Autodesk Inventor part; units mm, degrees
ref_plane "YZ Plane" through (0, 0, 0) normal (1, 0, 0) x (0, 1, 0)
ref_plane "XZ Plane" through (0, 0, 0) normal (0, 1, 0) x (-1, 0, 0)
ref_plane "XY Plane" through (0, 0, 0) normal (0, 0, 1) x (1, 0, 0)
sketch "Sketch1" plane through (0, 0, 0) normal (0, 0, 1) x (1, 0, 0)
  line L0 (9.525, -12.7) -> (-9.525, -12.7)
  line L1 (-9.525, -12.7) -> (-9.525, 12.7)
  line L2 (-9.525, 12.7) -> (9.525, 12.7)
  line L3 (9.525, 12.7) -> (9.525, -12.7)
  line L4 (9.525, -12.7) -> (-9.525, 12.7) construction
  line L5 (-9.525, -12.7) -> (9.525, 12.7) construction
  line L6 (-9.525, 12.7) -> (0, 12.7)
  line L7 (0, 12.7) -> (0, -50.8)
  line L8 (0, -50.8) -> (-9.525, -50.8)
  line L9 (-9.525, -50.8) -> (-9.525, 12.7)
  line L10 (-9.525, -50.8) -> (9.525, -43.8664)
  line L11 (-9.525, -50.8) -> (10.7476, -50.8) construction
  line L12 (9.525, -43.8664) -> (0, -35.8739)
  point P0 (0, 0)
  point P1 (0, -12.7)
  dimension "d0" = 19.05
  dimension "d1" = 25.4
  dimension "d2" = 63.5
  dimension "d3" = 20
  dimension "d4" = 60
extrude "Extrusion1" add sketch "Sketch1" along normal blind 3.175 contours L0 L7 L2 L3 | L7 L10 L9 L0 | L0 L1 L2 L7 | L12 L10 L7
sketch "Sketch2" plane through (0, 0, 3.175) normal (0, 0, 1) x (1, 0, 0)
  line L0 (-9.525, 12.7) -> (-9.525, -50.8) construction
  line L1 (-9.525, 0) -> (9.525, 0) construction
  line L2 (9.525, -12.7) -> (9.525, 12.7) construction
  line L3 (9.525, 12.7) -> (-9.525, 12.7) construction
  line L4 (0, -35.8739) -> (0, -12.7) construction
  line L5 (0, 12.7) -> (0, -12.7) construction
  circle A0 centre (3.175, 6.35) radius 1.5875
  circle A1 centre (3.175, -6.35) radius 1.5875
  circle A2 centre (-3.175, -6.35) radius 1.5875
  circle A3 centre (-3.175, 6.35) radius 1.5875
  line L6 (0, -12.7) -> (9.525, -12.7)
  point P0 (0, 0)
  dimension "d7" = 3.175
  dimension "d8" = 3.175
  dimension "d9" = 3.175
  dimension "d10" = 3.175
  dimension "d11" = 6.35
  dimension "d12" = 6.35
  dimension "d13" = 6.35
  dimension "d14" = 6.35
  dimension "d15" = 6.35
  dimension "d16" = 6.35
  dimension "d17" = 6.35
  dimension "d18" = 6.35
  dimension "d19" = 12.7
extrude "Extrusion2" cut sketch "Sketch2" against normal through all
fillet "Fillet1" radius 3.175 2 edges at (-9.525, -50.8, 1.5875) (0, -12.7, 1.5875)
fillet "Fillet2" radius 1.651 2 edges at (9.525, -43.8664, 1.5875) (0, -35.8739, 1.5875)
properties part number "CS_Climb_Hooks"
Geometry: final body of the model. Coordinates: model frame, mm. A direction names the side the tool comes from. Coordinates: 2 decimals unless noted, no trailing zeros. Order: outer loops, then holes, each group sorted by start corner. A loop starts at its lowest first (then second) coordinate and runs counter-clockwise, first axis right, second up. Notation, with made-up numbers: (25.5, 89.5) -> (46.5, 89.5) arc R33 cw to (46.5, 121.5) -> close; hole circle Ø5 at (-12, 72.25). An arc over 180 degrees is marked (long way). Write each question's results on one line, items separated by ' | '. Start each with the question number.
1) Set-up query: faces 1 (the cylindrical face through (-2.442, 4.942, 1.61)), 2 (the cylindrical face through (0.15, -35.79, 1.61)). Return all of +Z, -Z, +X, -X, +Y, -Y with unobstructed straight access to the full face (end or side cutting, diameter ignored); none if empty.
2) Material intervals for line 1 along Y through (x, z) = (2.5, 1.6); line 2 along X through (y, z) = (6, 0.6) (3 decimals); line 3 along X through (y, z) = (-20.5, 1.6) (3 decimals), sorted ascending.
3) Cut plane A-A, the plane z = 1.35. State how many separate pieces and enclosed holes the cut face has, and give its area (3 significant figures).
4) Cut plane B-B, the plane y = -6.35. Output: boundary loops of the cut face in (x, z) (1 decimal).
5) Mould query, pull axis X, two halves, no side actions, for faces 3 (the cylindrical face through (1.92, -7.32, 1.61)), 4 (the flat face through (-9.525, -17, 2)), 5 (the cylindrical face through (7.895, -43.604, 1.61)), 6 (the flat face through (0, 12.7, 2)). Classes: released by +X, released by -X, zero draft, split by the parting line, or undercut.
6) Cut plane D-D, the plane y = -43.5. Output: boundary loops of the cut face in (x, z) (3 decimals), and give its area (3 significant figures).
7) Cut plane C-C, the plane y = -17. Output: boundary loops of the cut face in (x, z) (3 decimals).
8) First-contact query: pin 1 (1 mm diameter, centred on x = -2, z = 2, fed in from -Y); pin 2 (2.5 mm diameter, centred on x = -3.175, y = 6.35, fed in from +Z); pin 3 (1.6 mm diameter, centred on x = 5, z = 1, fed in from -Y). Flat tips, straight axial feed; report the tip coordinate or a pass-through.
Checks:
1) face 1: +Z, -Z | face 2: +Z, -Z, +X
2) line 1: -46.42 to -37.97, -12.77 to -7.79, -4.91 to 4.91, 7.79 to 12.7 | line 2: -9.525 to -4.723, -1.627 to 1.627, 4.723 to 9.525 | line 3: -9.525 to 0
3) separate pieces: 1 | enclosed holes: 4 | area: 849 mm^2
4) outline: (-9.5, 0) -> (-4.8, 0) -> (-4.8, 3.2) -> (-9.5, 3.2) -> close; (-1.6, 0) -> (1.6, 0) -> (1.6, 3.2) -> (-1.6, 3.2) -> close; (4.8, 0) -> (9.5, 0) -> (9.5, 3.2) -> (4.8, 3.2) -> close
5) face 3: undercut | face 4: released by -X | face 5: released by +X | face 6: zero draft
6) outline: (-9.525, 0) -> (7.911, 0) -> (7.911, 3.175) -> (-9.525, 3.175) -> close | area: 55.4 mm^2
7) outline: (-9.525, 0) -> (0, 0) -> (0, 3.175) -> (-9.525, 3.175) -> close
8) pin 1: y = -48.24 | pin 2: through | pin 3: y = -45.8
